from build123d import *

# Parameters (mm, degrees)
SKETCH1_R           = 3.975
BOSS_EXTRUDE1_DEPTH = 30
BOSS_EXTRUDE2_DEPTH = 30
CHAMFER2_SIZE       = 0.5


with BuildPart() as part:
    # Sketch1 → Boss-Extrude1 (new body)
    with BuildSketch(Plane.XY):
        Circle(SKETCH1_R)
    extrude(amount=BOSS_EXTRUDE1_DEPTH)

    # Sketch2 → Boss-Extrude2 (add)
    with BuildSketch(Plane.XY.offset(30)):
        Polygon((3.95669873, 0), (1.978349365, 3.426601615), (-1.978349365, 3.426601615), (-3.95669873, 0), (-1.978349365, -3.426601615), (1.978349365, -3.426601615), align=None)
    extrude(amount=BOSS_EXTRUDE2_DEPTH)

    # Chamfer2
    chamfer2_edges = [part.edges().sort_by_distance(p)[0] for p in [
        (2.967524047, -1.713300808, 60),
        (2.967524047, 1.713300808, 60),
        (0, 3.426601615, 60),
        (-2.967524047, 1.713300808, 60),
        (-2.967524047, -1.713300808, 60),
        (0, -3.426601615, 60),
    ]]
    chamfer(chamfer2_edges, length=CHAMFER2_SIZE)


solid = part.part
Verification items for the finished model (mm, model axes). A direction names the side the tool comes from. Coordinates: 2 decimals unless noted, no trailing zeros. Write each loop counter-clockwise with the first axis right and the second up, starting at its lowest first coordinate (ties: lowest second). Pieces come first, ordered by that corner, then holes. Notation, with made-up numbers: M 65.25,19 L 80.25,19 A15 cw 80.25,48 Z; hole C -2.75,82 d8. An arc over 180 degrees is marked long. Use a Markdown table: item, result.
Q1. Go/stop test with flat-tipped pins: P1, Ø4, axis at x = -0.5, z = 9.5, coming from the +Y side (3 decimals); P2, Ø1.2, axis at x = 0, z = 50, coming from the +Y side; P3, Ø4, axis at x = -2.5, z = 29.5, coming from the +Y side; P4, Ø4.5, axis at x = 0, z = 41.5, coming from the -Y side. Record where each tip stops, or that it passes through.
Reply:
| item | result |
|---|---|
| P1 | stops at y = 3.975 |
| P2 | stops at y = 3.43 |
| P3 | stops at y = 3.94 |
| P4 | stops at y = -3.43 |
Q2. Thickness scan on line 1 (Z direction, x = -0.5, y = 3.75); line 2 (Y direction, x = 0.5, z = 50.5); line 3 (X direction, y = -1.75, z = 22.5). Record the ranges inside material, lowest first.
Reply:
| item | result |
|---|---|
| line 1 | z = 0 to 30 |
| line 2 | y = -3.43 to 3.43 |
| line 3 | x = -3.57 to 3.57 |
Q3. Sectioned sample at B-B, the plane z = 35.5. Record the boundary of the cut face in (x, y), plus the area to 3 significant figures.
Reply:
| item | result |
|---|---|
| outline | M -3.96,0 L -1.98,-3.43 L 1.98,-3.43 L 3.96,0 L 1.98,3.43 L -1.98,3.43 Z |
| area | 40.7 mm² |
Q4. Set-up check for faces 1 (the face through (0, 3.427, 45)), 2 (the face through (0, -3.427, 45)), 3 (the face through (-2.98, -1.69, 44.54)): record each of +Z, -Z, +X, -X, +Y, -Y from which the full face is reachable in a straight line by a thin tool's end or side.
Reply:
| item | result |
|---|---|
| face 1 | +Z, +X, -X, +Y |
| face 2 | +Z, +X, -X, -Y |
| face 3 | +Z, -X, -Y |
Q5. Sectioned sample at A-A, the plane x = 0. Record the boundary of the cut face in (y, z) (3 decimals).
Reply:
| item | result |
|---|---|
| outline | M -3.975,0 L 3.975,0 L 3.975,30 L 3.427,30 L 3.427,59.5 L 2.927,60 L -2.927,60 L -3.427,59.5 L -3.427,30 L -3.975,30 Z |
Q6. Sectioned sample at C-C, the plane y = 2. Record the boundary of the cut face in (x, z).
Reply:
| item | result |
|---|---|
| outline | M -3.44,0 L 3.44,0 L 3.44,30 L 2.8,30 L 2.8,59.5 L 2.22,60 L -2.22,60 L -2.8,59.5 L -2.8,30 L -3.44,30 Z |
